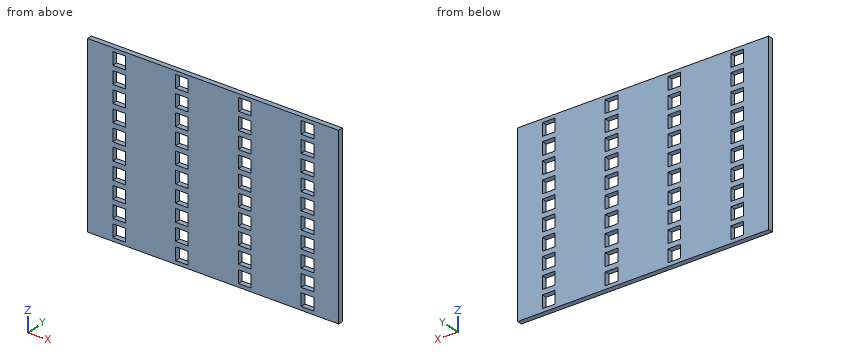
```python
from build123d import *

# Parameters (mm, degrees)
SKETCH1_W           = 100
SKETCH1_H           = 70
BOSS_EXTRUDE1_DEPTH = 2
SKETCH2_W           = 5
SKETCH2_H           = 5
CUT_EXTRUDE1_DEPTH  = 10


with BuildPart() as part:
    # Sketch1 → Boss-Extrude1 (new body)
    with BuildSketch(Plane(origin=(0, 0, 0), x_dir=(1, 0, 0), z_dir=(0, 1, 0))):
        with Locations((-22.5, 23.020833333)):
            Rectangle(SKETCH1_W, SKETCH1_H)
    extrude(amount=BOSS_EXTRUDE1_DEPTH)

    # Sketch2 → Cut-Extrude1 (cut)
    with BuildSketch(Plane(origin=(0, 2, 0), x_dir=(1, 0, 0), z_dir=(0, 1, 0))):
        with Locations((-34.922189654, 54.160833333)):
            Rectangle(SKETCH2_W, SKETCH2_H)
        with Locations((-59.922189654, 54.160833333)):
            Rectangle(SKETCH2_W, SKETCH2_H)
        with Locations((-9.922189654, 54.160833333)):
            Rectangle(SKETCH2_W, SKETCH2_H)
        with Locations((15.077810346, 54.160833333)):
            Rectangle(SKETCH2_W, SKETCH2_H)
        with Locations((-34.922189654, 47.240833333)):
            Rectangle(SKETCH2_W, SKETCH2_H)
        with Locations((-9.922189654, 47.240833333)):
            Rectangle(SKETCH2_W, SKETCH2_H)
        with Locations((15.077810346, 47.240833333)):
            Rectangle(SKETCH2_W, SKETCH2_H)
        with Locations((-34.922189654, 40.320833333)):
            Rectangle(SKETCH2_W, SKETCH2_H)
        with Locations((-9.922189654, 40.320833333)):
            Rectangle(SKETCH2_W, SKETCH2_H)
        with Locations((15.077810346, 40.320833333)):
            Rectangle(SKETCH2_W, SKETCH2_H)
        with Locations((-34.922189654, 33.400833333)):
            Rectangle(SKETCH2_W, SKETCH2_H)
        with Locations((-9.922189654, 33.400833333)):
            Rectangle(SKETCH2_W, SKETCH2_H)
        with Locations((15.077810346, 33.400833333)):
            Rectangle(SKETCH2_W, SKETCH2_H)
        with Locations((-34.922189654, 26.480833333)):
            Rectangle(SKETCH2_W, SKETCH2_H)
        with Locations((-9.922189654, 26.480833333)):
            Rectangle(SKETCH2_W, SKETCH2_H)
        with Locations((15.077810346, 26.480833333)):
            Rectangle(SKETCH2_W, SKETCH2_H)
        with Locations((-34.922189654, 19.560833333)):
            Rectangle(SKETCH2_W, SKETCH2_H)
        with Locations((-9.922189654, 19.560833333)):
            Rectangle(SKETCH2_W, SKETCH2_H)
        with Locations((15.077810346, 19.560833333)):
            Rectangle(SKETCH2_W, SKETCH2_H)
        with Locations((-34.922189654, 12.640833333)):
            Rectangle(SKETCH2_W, SKETCH2_H)
        with Locations((-9.922189654, 12.640833333)):
            Rectangle(SKETCH2_W, SKETCH2_H)
        with Locations((15.077810346, 12.640833333)):
            Rectangle(SKETCH2_W, SKETCH2_H)
        with Locations((-34.922189654, 5.720833333)):
            Rectangle(SKETCH2_W, SKETCH2_H)
        with Locations((-9.922189654, 5.720833333)):
            Rectangle(SKETCH2_W, SKETCH2_H)
        with Locations((15.077810346, 5.720833333)):
            Rectangle(SKETCH2_W, SKETCH2_H)
        with Locations((-34.922189654, -1.199166667)):
            Rectangle(SKETCH2_W, SKETCH2_H)
        with Locations((-9.922189654, -1.199166667)):
            Rectangle(SKETCH2_W, SKETCH2_H)
        with Locations((15.077810346, -1.199166667)):
            Rectangle(SKETCH2_W, SKETCH2_H)
        with Locations((-34.922189654, -8.119166667)):
            Rectangle(SKETCH2_W, SKETCH2_H)
        with Locations((-9.922189654, -8.119166667)):
            Rectangle(SKETCH2_W, SKETCH2_H)
        with Locations((15.077810346, -8.119166667)):
            Rectangle(SKETCH2_W, SKETCH2_H)
        with Locations((-59.922189654, 47.240833333)):
            Rectangle(SKETCH2_W, SKETCH2_H)
        with Locations((-59.922189654, 40.320833333)):
            Rectangle(SKETCH2_W, SKETCH2_H)
        with Locations((-59.922189654, 33.400833333)):
            Rectangle(SKETCH2_W, SKETCH2_H)
        with Locations((-59.922189654, 26.480833333)):
            Rectangle(SKETCH2_W, SKETCH2_H)
        with Locations((-59.922189654, 19.560833333)):
            Rectangle(SKETCH2_W, SKETCH2_H)
        with Locations((-59.922189654, 12.640833333)):
            Rectangle(SKETCH2_W, SKETCH2_H)
        with Locations((-59.922189654, 5.720833333)):
            Rectangle(SKETCH2_W, SKETCH2_H)
        with Locations((-59.922189654, -1.199166667)):
            Rectangle(SKETCH2_W, SKETCH2_H)
        with Locations((-59.922189654, -8.119166667)):
            Rectangle(SKETCH2_W, SKETCH2_H)
    extrude(amount=-CUT_EXTRUDE1_DEPTH, mode=Mode.SUBTRACT)


solid = part.part
```
The model under review builds one solid part; all positions refer to its coordinate system, in mm. Give positions to 0.01 mm unless a question says otherwise; leave off trailing zeros. Loops run counter-clockwise (first coordinate to the right, second up) from the corner with the lowest first, then second, coordinate; pieces in that order, holes last. Notation, with made-up numbers: (-2.75, 67) - (5.25, 67) arc R16 cw to (5.25, 92) - close; hole circle Ø8 at (57.25, -38.5). An arc over 180 degrees is marked (long way). Answer as a JSON object with one key per item and string values.
Q1. To check wall thickness, follow line 1 along X through (y, z) = (1, -39.5). State the ranges of the line that lie inside material, in increasing order.
Worked out:
{"line 1": "x = -72.5 to -62.42, -57.42 to -37.42, -32.42 to -12.42, -7.42 to 12.58, 17.58 to 27.5"}
Q2. Add section A-A on z = -25.5. State the section outline as (x, y) points.
Worked out:
{"outline": "(-72.5, 0) - (-62.42, 0) - (-62.42, 2) - (-72.5, 2) - close; (-57.42, 0) - (-37.42, 0) - (-37.42, 2) - (-57.42, 2) - close; (-32.42, 0) - (-12.42, 0) - (-12.42, 2) - (-32.42, 2) - close; (-7.42, 0) - (12.58, 0) - (12.58, 2) - (-7.42, 2) - close; (17.58, 0) - (27.5, 0) - (27.5, 2) - (17.58, 2) - close"}
Q3. Insertion check: pin 1 (3 mm diameter, centred on x = 5, z = -18, fed in from -Y). The pin has a flat end and moves straight along its axis. Give the tip position at first contact, or say it passes through.
Worked out:
{"pin 1": "stops at y = 0"}
Q4. Add section B-B on x = -34. Count the separate pieces of the cut face and the enclosed holes in it, plus the area to 3 significant figures.
Worked out:
{"separate pieces": "11", "enclosed holes": "0", "area": "40.0 mm^2"}
